Autodesk Inventor part; units mm, degrees
ref_plane "YZ Plane" through (0, 0, 0) normal (1, 0, 0) x (0, 1, 0)
ref_plane "XZ Plane" through (0, 0, 0) normal (0, 1, 0) x (-1, 0, 0)
ref_plane "XY Plane" through (0, 0, 0) normal (0, 0, 1) x (1, 0, 0)
sketch "Sketch1" plane through (0, 0, 0) normal (0, 1, 0) x (-1, 0, 0)
  line L0 (53.5, 38) -> (40.125, 14.25)
  line L1 (40.125, 14.25) -> (0, 0)
  line L2 (1.6733, -4.7117) -> (43.5628, 10.165)
  line L3 (43.5628, 10.165) -> (57.8567, 35.5465)
  line L4 (-1.6733, 4.7117) -> (36.6872, 18.335)
  line L5 (36.6872, 18.335) -> (49.1433, 40.4535)
  arc A0 (-1.6733, 4.7117) -> (1.6733, -4.7117) centre (0, 0) ccw
  arc A1 (57.8567, 35.5465) -> (49.1433, 40.4535) centre (53.5, 38) ccw
  dimension "d0" = 5
  dimension "d1" = 5
  dimension "d2" = 40.7078
  dimension "d3" = 5
  dimension "d4" = 25.3847
  dimension "d5" = 29.1297
  dimension "d6" = 53.5
extrude "Extrusion1" add sketch "Sketch1" along normal mid plane 5
sketch "Sketch2" plane through (0, 2.5, 0) normal (0, 1, 0) x (1, 0, 0)
  point P0 (0, 0)
  point P1 (0, 0)
hole "Hole1" at (0, 2.5, 0) direction (0, -1, 0) diameter 3.302 depth 12.3 tip angle 118
sketch "Sketch3" plane through (0, 2.5, 0) normal (0, 1, 0) x (1, 0, 0)
  line L0 (-50.6525, -39.6036) -> (-48.6527, -39.5822)
  line L1 (-48.6527, -39.5822) -> (-49.634, -41.3248)
  line L2 (-49.634, -41.3248) -> (-50.6525, -39.6036)
  arc A0 (-57.8567, -35.5465) -> (-49.1433, -40.4535) centre (-53.5, -38) ccw
  line L3 (-49.1433, -40.4535) -> (-36.6872, -18.335)
  line L4 (-36.6872, -18.335) -> (-49.1433, -40.4535)
  line L5 (-49.1433, -40.4535) -> (-57.8567, -35.5465)
  line L6 (-51.4829, -40.5712) -> (-49.6271, -41.3167)
  line L7 (-49.6271, -41.3167) -> (-51.2007, -42.5512)
  line L8 (-51.2007, -42.5512) -> (-51.4829, -40.5712)
  line L9 (-52.6204, -41.1474) -> (-51.1912, -42.5463)
  line L10 (-51.1912, -42.5463) -> (-53.1174, -43.0846)
  line L11 (-53.1174, -43.0846) -> (-52.6204, -41.1474)
  line L12 (-53.8918, -41.2444) -> (-53.1067, -43.0838)
  line L13 (-53.1067, -43.0838) -> (-55.0923, -42.844)
  line L14 (-55.0923, -42.844) -> (-53.8918, -41.2444)
  line L15 (-55.1036, -40.8475) -> (-55.0822, -42.8473)
  line L16 (-55.0822, -42.8473) -> (-56.8248, -41.866)
  line L17 (-56.8248, -41.866) -> (-55.1036, -40.8475)
  line L18 (-56.0712, -40.0171) -> (-56.8167, -41.8729)
  line L19 (-56.8167, -41.8729) -> (-58.0512, -40.2993)
  line L20 (-58.0512, -40.2993) -> (-56.0712, -40.0171)
  line L21 (-56.6474, -38.8796) -> (-58.0463, -40.3088)
  line L22 (-58.0463, -40.3088) -> (-58.5846, -38.3826)
  line L23 (-58.5846, -38.3826) -> (-56.6474, -38.8796)
  line L24 (-56.7444, -37.6082) -> (-58.5838, -38.3933)
  line L25 (-58.5838, -38.3933) -> (-58.344, -36.4077)
  line L26 (-58.344, -36.4077) -> (-56.7444, -37.6082)
  line L27 (-56.3475, -36.3964) -> (-58.3473, -36.4178)
  line L28 (-58.3473, -36.4178) -> (-57.366, -34.6752)
  line L29 (-57.366, -34.6752) -> (-56.3475, -36.3964)
  point P0 (0, 0)
  point P1 (-49.6464, -40.1702)
  point P2 (-50.7702, -41.4797)
  point P3 (-52.3096, -42.2594)
  point P4 (-54.0303, -42.3907)
  point P5 (-55.6702, -41.8536)
  point P6 (-56.9797, -40.7298)
  point P7 (-57.7594, -39.1904)
  point P8 (-57.8907, -37.4697)
  point P9 (-57.3536, -35.8298)
  dimension "d16" = 2
  dimension "d19" = 180
extrude "Extrusion2" cut sketch "Sketch3" against normal through all contours L5 A0 L2 | L0 L1 L5 | A0 L1 L2 | L27 A0 L5 | L5 L28 L29 | L7 A0 L6 | A0 L8 L6 | A0 L27 L28 | L7 L8 A0 | L26 A0 L25 | L26 L24 A0 | L10 A0 L9 | A0 L24 L25 | A0 L11 L9 | L10 L11 A0 | L23 A0 L22 | L13 A0 L12 | L23 L21 A0 | A0 L21 L22 | A0 L14 L12 | L13 L14 A0 | L20 A0 L19 | L16 A0 L15 | L20 L18 A0 | A0 L18 L19 | A0 L17 L15 | L16 L17 A0
properties part number "Finger"
For this review, take the finished solid that the model builds, in its own axes (mm). Round coordinates to 2 decimals unless told otherwise and drop trailing zeros. Write each loop counter-clockwise with the first axis right and the second up, starting at its lowest first coordinate (ties: lowest second). Pieces come first, ordered by that corner, then holes. Notation, with made-up numbers: (69, -18.5) -> (116, -18.5) arc R24 ccw to (116, 17.5) -> close; hole circle Ø5 at (-22, 59). An arc over 180 degrees is marked (long way). Use one line per item in the form item = value.
Q1. Clearance check with flat-ended pins moving along their axes: pin 1 Ø2 at (x, y) = (-48, 0) entering from -Z; pin 2 Ø2 at (x, y) = (-51, 0.5) entering from +Z. State where each tip first meets the part, or that it passes through.
Resolved:
pin_1 = 16.27
pin_2 = 42.47
Q2. Consider section C-C (x = 0). State the section outline as (y, z) points, then the cut area to 3 significant figures.
Resolved:
outline = (-2.5, -5) -> (2.5, -5) -> (2.5, -1.65) -> (-2.5, -1.65) -> close; (-2.5, 1.65) -> (2.5, 1.65) -> (2.5, 5.31) -> (-2.5, 5.31) -> close
area = 35.0 mm²
Q3. The part is to be moulded in two halves that separate along X. For faces 1 (the flat face through (-29, -2.5, 14)), 2 (the flat face through (-53.525, 0.035, 42.104)), 3 (the flat face through (-22.32, -0.04, 2.62)), say which applies: released by +X, released by -X, zero draft, split by the parting line, or undercut.
Resolved:
face_1 = zero draft
face_2 = undercut
face_3 = released by -X
Q4. To check wall thickness, follow probe 1 along Z at (x, y) = (0, 0.15); probe 2 along Z at (x, y) = (-26.5, 1.85); probe 3 along Z at (x, y) = (-54.5, -1.15). State the ranges of each line that lie inside material, in increasing order. Write a range as from..to.
Resolved:
probe_1 = -5..-1.65, 1.65..5.31
probe_2 = 4.11..14.72
probe_3 = 29.59..42.05
Q5. Consider section D-D (z = 25). State the section outline as (x, y) points, then the cut area to 3 significant figures.
Resolved:
outline = (-51.92, -2.5) -> (-40.44, -2.5) -> (-40.44, 2.5) -> (-51.92, 2.5) -> close
area = 57.4 mm²
Q6. Consider section A-A (z = 0). State the section outline as (x, y) points, then the cut area to 3 significant figures.
Resolved:
outline = (-14.94, -2.5) -> (-1.65, -2.5) -> (-1.65, 2.5) -> (-14.94, 2.5) -> close; (1.65, -2.5) -> (5, -2.5) -> (5, 2.5) -> (1.65, 2.5) -> close
area = 83.2 mm²
